Autodesk Fusion 360 part; units mm, degrees
sketch "Boceto2" plane through (0, 0, 0) normal (0, 1, 0) x (1, 0, 0)
  circle A0 centre (0, 0) radius 6.6
  dimension "d1" = 13.2
ref_plane "PlanoDeObra1" through (0, 5, 0) normal (0, 1, 0) x (1, 0, 0)
sketch "Boceto3" plane through (0, 5, 0) normal (0, 1, 0) x (1, 0, 0)
  circle A0 centre (0, 0) radius 9.4
  dimension "d3" = 18.8
ref_plane "PlanoDeObra2" through (0, 34.5, 0) normal (0, 1, 0) x (1, 0, 0)
sketch "Boceto4" plane through (0, 34.5, 0) normal (0, 1, 0) x (1, 0, 0)
  circle A0 centre (0, 0) radius 10.65
  dimension "d5" = 21.3
loft "Solevación1" add profiles "Boceto2", "Boceto3" section 1 section 2
loft "Solevación2" add profiles "Boceto4" section 1 face at (2.1836, 5, -0.9236) section 2
ref_plane "PlanoDeObra3" through (0, 101.7, 0) normal (0, 1, 0) x (0, 0, 1)
sketch "Boceto5" plane through (0, 101.7, 0) normal (0, 1, 0) x (1, 0, 0)
  circle A0 centre (0, 0) radius 9.25
  dimension "d7" = 18.5
loft "Solevación3" add profiles "Boceto5" section 1 face at (-2.6023, 34.5, 4.1946) section 2
ref_plane "PlanoDeObra4" through (0, 104.5, 0) normal (0, 1, 0) x (0, 0, 1)
sketch "Boceto6" plane through (0, 104.5, 0) normal (0, 1, 0) x (1, 0, 0)
  circle A0 centre (0, 0) radius 8.15
  dimension "d9" = 16.3
ref_plane "PlanoDeObra5" through (0, 109.7, 0) normal (0, 1, 0) x (1, 0, 0)
sketch "Boceto7" plane through (0, 109.7, 0) normal (0, 1, 0) x (1, 0, 0)
  circle A0 centre (0, 0) radius 6.55
  dimension "d11" = 13.1
ref_plane "PlanoDeObra6" through (0, 120.9, 0) normal (0, 1, 0) x (1, 0, 0)
sketch "Boceto8" plane through (0, 120.9, 0) normal (0, 1, 0) x (1, 0, 0)
  circle A0 centre (0, 0) radius 4
  dimension "d13" = 8
loft "Solevación4" add profiles "Boceto6" section 1 face at (-2.5312, 101.7, -3.8946) section 2
extrude "Extruir1" add sketch "Boceto7" against normal blind 5.2
extrude "Extruir2" add sketch "Boceto8" against normal blind 11.2
fillet "Empalme1" radius 1.5 1 edges at (-6.1067, 104.5, -2.3686)
chamfer "Chaflán1" distance 2.55 distance2 4 1 edges at (-3.7293, 109.7, -1.4465) measured on face at (5.6756, 109.7, 0.3254)
ref_plane "PlanoDeObra7" through (0, 126.7, 0) normal (0, -1, 0) x (0, 0, -1)
sketch "Boceto9" plane through (0, 120.9, 0) normal (0, 1, 0) x (-1, 0, 0)
  circle A0 centre (0, 0) radius 4
  circle A1 centre (0, 0) radius 2.6
  dimension "d23" = 5.2
extrude "Extruir3" add sketch "Boceto9" along normal up to surface (5.8 mm away) contours A1
fillet "Empalme2" radius 2.47 1 edges at (2.4241, 126.7, -0.9402)
equation "d4 = 25.5 mm + 4 mm"
equation "d27 = ( ( 5.2 / 2 ) * 0.95 ) * 1 mm"
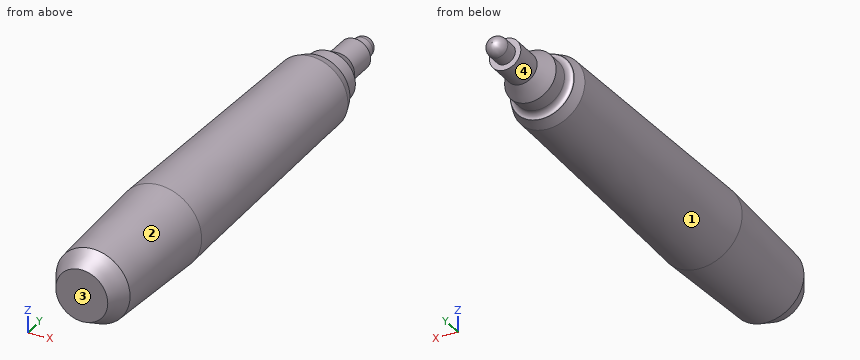
For this review, take the finished solid that the model builds, in its own axes (mm). Face numbers are marked on the shaded views. A direction names the side the tool comes from. Round coordinates to 2 decimals unless told otherwise and drop trailing zeros. Order: outer loops, then holes, each group sorted by start corner. A loop starts at its lowest first (then second) coordinate and runs counter-clockwise, first axis right, second up. Notation, with made-up numbers: M -23,-16.5 L 23,-16.5 A17 cw 23,-11.5 Z; hole C 49.25,34.25 d7. An arc over 180 degrees is marked long. Write each question's results on one line, items separated by ' | '. Start each with the question number.
1. Tool access review of the marked faces 1 and 2: name each direction out of +Z, -Z, +X, -X, +Y, -Y from which nothing blocks a thin tool from reaching the whole face with its end or side.
2. To check wall thickness, follow L1, parallel to Z at x = 0.5, y = 109.5; L2, parallel to Y at x = 1, z = -2.5; L3, parallel to X at y = 84.5, z = -0.75. State the ranges of each line that lie inside material, in increasing order. Write a range as [from, to].
3. Add section B-B (y = 43). State the section outline as (x, z) points, then the cut area to 3 significant figures.
4. Clearance check with flat-ended pins moving along their axes: pin 1 Ø5 at (y, z) = (89, -6.5) entering from +X; pin 2 Ø3 at (y, z) = (27, 0.5) entering from +X; pin 3 Ø5 at (y, z) = (24.5, -7) entering from +X. State where each tip first meets the part, or that it passes through.
5. Add section A-A (y = 66). State the section outline as (x, z) points.
6. Draft analysis for pull direction X (two halves, no side actions). For the marked faces 3 and 4, state which applies: pulls with the +X half, pulls with the -X half, needs draft (parallel to the pull), parting line crosses it, or undercut.
Output values:
1) face 1: +Y | face 2: -Y
2) L1: [-6.53, 6.53] | L2: [0, 120.9] | L3: [-9.58, 9.58]
3) outline: C 0,0 d20.95 | area: 345 mm^2
4) pin 1: x = 8.63 | pin 2: x = 10.39 | pin 3: x = 9.19
5) outline: C 0,0 d19.99
6) face 3: needs draft | face 4: parting line crosses it
